Geometry check sheet. Reference: the model listing, model coordinates, mm. A direction names the side the tool comes from. Coordinates: 2 decimals unless noted, no trailing zeros. Use CSV: the item, a comma, the result in double quotes.
Autodesk Inventor part; units mm, degrees
ref_plane "YZ Plane" through (0, 0, 0) normal (1, 0, 0) x (0, 1, 0)
ref_plane "XZ Plane" through (0, 0, 0) normal (0, 1, 0) x (-1, 0, 0)
ref_plane "XY Plane" through (0, 0, 0) normal (0, 0, 1) x (1, 0, 0)
sketch "スケッチ2" plane through (0, 0, 0) normal (1, 0, 0) x (0, 1, 0)
  line L0 (0, 0) -> (-84.4498, 0)
  line L1 (-84.4498, -20) -> (1.7498, -20)
  line L2 (0, 0) -> (83.1668, 14.6646)
  line L3 (86.6398, -5.0316) -> (1.7498, -20)
  arc A0 (87.251, 14.537) -> (83.1668, 14.6646) centre (84.9033, 4.8165) ccw
  arc A1 (86.6398, -5.0316) -> (90.434, -3.5148) centre (84.9033, 4.8165) ccw
  arc A2 (-88.4498, -19.1652) -> (-84.4498, -20) centre (-84.4498, -10) ccw
  arc A3 (-84.4498, 0) -> (-88.4498, -0.8348) centre (-84.4498, -10) ccw
  arc A4 (-84.4498, -14) -> (-84.4498, -6) centre (-84.4498, -10) ccw
  line L4 (-84.4498, -6) -> (-88.4498, -6)
  line L5 (-84.4498, -14) -> (-88.4498, -14)
  line L6 (-88.4498, -0.8348) -> (-88.4498, -6)
  line L7 (-88.4498, -14) -> (-88.4498, -19.1652)
  line L8 (87.251, 14.537) -> (88.1479, 9.4503)
  line L9 (89.5371, 1.5718) -> (90.434, -3.5148)
  line L10 (1.7498, -20) -> (0, 0)
  line L11 (88.1479, 9.4503) -> (89.5371, 1.5718)
  dimension "d21" = 20
  dimension "d22" = 10
  dimension "d23" = 170
  dimension "d27" = 10
  dimension "d31" = 8
  dimension "d33" = 4
  dimension "d35" = 4
  dimension "d36" = 170
  dimension "d139" = 20
extrude "押し出し1" add sketch "スケッチ2" along normal blind 2
sketch "スケッチ4" plane through (0, 0, 0) normal (-1, 0, 0) x (0, 0, 1)
  line L0 (-20, 1.7498) -> (-5.0316, 86.6398)
  line L1 (-20, -84.4498) -> (-20, 1.7498)
  circle A0 centre (-17, -18.5891) radius 1
  circle A1 centre (-13.5138, 21.2587) radius 1
  line L2 (-17, -18.5891) -> (-13.5138, 21.2587)
  line L3 (-20, 1.7498) -> (0, 0)
  dimension "d57" = 2
  dimension "d59" = 40
  dimension "d60" = 175
  dimension "d61" = 3
  dimension "d62" = 3
hole "穴2" at (0, -18.5891, -17) at (0, 21.2587, -13.5138) direction (1, 0, 0) diameter 1.6 end through all
sketch "スケッチ6" plane through (2, 0, 0) normal (1, 0, 0) x (0, 0, -1)
  line L0 (20, 1.7498) -> (5.0316, 86.6398)
  arc A0 (5.0316, 86.6398) -> (3.5148, 90.434) centre (-4.8165, 84.9033) ccw
  line L1 (3.5148, 90.434) -> (-14.537, 87.251)
  arc A1 (-14.537, 87.251) -> (-14.6646, 83.1668) centre (-4.8165, 84.9033) ccw
  line L2 (-14.6646, 83.1668) -> (0, 0)
  line L3 (-9.3978, 53.2975) -> (-12.6117, 57.1277)
  line L4 (-14.537, 87.251) -> (-17.8212, 86.6719)
  line L5 (-17.8212, 86.6719) -> (-12.6117, 57.1277)
  line L6 (3.5148, 90.434) -> (6.799, 91.0131)
  line L7 (6.799, 91.0131) -> (12.0085, 61.4689)
  line L8 (12.0085, 61.4689) -> (10.2984, 56.7704)
  dimension "d75" = 150
  dimension "d76" = 150
  dimension "d77" = 2.5
  dimension "d78" = 2.5
  dimension "d79" = 30
extrude "押し出し2" add sketch "スケッチ6" against normal blind 2
sketch "スケッチ5" plane through (2, 0, 0) normal (1, 0, 0) x (0, 0, -1)
  line L0 (3.5148, 90.434) -> (-14.537, 87.251)
  circle A0 centre (-12.5213, 82.5293) radius 1.5
  circle A1 centre (3.2356, 85.3077) radius 1.5
  line L1 (-12.6117, 57.1277) -> (-17.8212, 86.6719)
  line L2 (-17.8212, 86.6719) -> (6.799, 91.0131)
  line L3 (6.799, 91.0131) -> (12.0085, 61.4689)
  line L4 (12.0085, 61.4689) -> (10.2984, 56.7704)
  line L5 (10.2984, 56.7704) -> (20, 1.7498)
  line L6 (20, 1.7498) -> (20, -84.4498)
  arc A2 (19.1652, -88.4498) -> (20, -84.4498) centre (10, -84.4498) ccw
  line L7 (19.1652, -88.4498) -> (14, -88.4498)
  line L8 (14, -88.4498) -> (14, -84.4498)
  arc A3 (14, -84.4498) -> (6, -84.4498) centre (10, -84.4498) ccw
  line L9 (6, -84.4498) -> (6, -88.4498)
  line L10 (6, -88.4498) -> (0.8348, -88.4498)
  arc A4 (0, -84.4498) -> (0.8348, -88.4498) centre (10, -84.4498) ccw
  line L11 (0, -84.4498) -> (0, 0)
  line L12 (0, 0) -> (-9.3978, 53.2975)
  line L13 (-9.3978, 53.2975) -> (-12.6117, 57.1277)
  circle A5 centre (17, -18.5891) radius 0.8
  circle A6 centre (13.5138, 21.2587) radius 0.8
  dimension "d70" = 5
  dimension "d71" = 5
  dimension "d72" = 3
  dimension "d114" = 16
  dimension "d123" = 4.5
hole "穴3" at (2, 82.5293, 12.5213) at (2, 85.3077, -3.2356) direction (-1, 0, 0) diameter 4 end through all
sketch "スケッチ7" plane through (2, 0, 0) normal (1, 0, 0) x (0, 0, -1)
  arc A0 (0, -84.4498) -> (0.8348, -88.4498) centre (10, -84.4498) ccw
  line L0 (0.8348, -88.4498) -> (6, -88.4498)
  circle A1 centre (3, -84.4498) radius 1
  dimension "d89" = 4
  dimension "d90" = 7
  dimension "d91" = 2
hole "穴4" at (2, -84.4498, -3) direction (-1, 0, 0) diameter 2 end through all
pattern_circular "円形状パターン3" count 5 over 180 about axis through (0, -84.4498, -10) along (-1, 0, 0) of "穴4"
sketch "スケッチ8" plane through (2, 0, 0) normal (1, 0, 0) x (0, 0, -1)
  line L0 (6.799, 91.0131) -> (-17.8212, 86.6719)
  line L1 (-17.8212, 86.6719) -> (-12.6117, 57.1277)
  circle A0 centre (-11.4794, 76.6205) radius 1.5
  circle A1 centre (4.2775, 79.3988) radius 1.5
  dimension "d102" = 11
  dimension "d103" = 11
  dimension "d104" = 16
  dimension "d105" = 4.5
  dimension "d106" = 3
hole "穴5" at (2, 76.6205, 11.4794) at (2, 79.3988, -4.2775) direction (-1, 0, 0) diameter 3.5 end through all
sketch "スケッチ11" plane through (2, 0, 0) normal (1, 0, 0) x (0, 0, -1)
  circle A0 centre (-11.4794, 76.6205) radius 1.75
  circle A1 centre (4.2775, 79.3988) radius 1.75
  line L0 (-17.8212, 86.6719) -> (-12.6117, 57.1277)
  circle A2 centre (-8.8747, 61.8483) radius 1.5
  circle A3 centre (6.8822, 64.6267) radius 1.5
  dimension "d124" = 3
  dimension "d126" = 16
  dimension "d127" = 15
  dimension "d128" = 4.5
  dimension "d130" = 15
hole "穴6" at (2, 61.8483, 8.8747) at (2, 64.6267, -6.8822) direction (-1, 0, 0) diameter 3.5 end through all
sketch "スケッチ13" plane through (2, 0, 0) normal (1, 0, 0) x (0, 0, -1)
  line L0 (0, 0) -> (0, -84.4498)
  line L1 (20, -84.4498) -> (20, 1.7498)
  line L2 (20, 1.7498) -> (10.2984, 56.7704)
  line L3 (6.799, 91.0131) -> (-17.8212, 86.6719)
  line L4 (-9.3978, 53.2975) -> (0, 0)
  line L5 (-3.8662, 44.9615) -> (9.2538, 39.6592)
  line L6 (9.2538, 39.6592) -> (6.6491, 54.4313)
  line L7 (6.6491, 54.4313) -> (-3.8662, 44.9615)
  line L8 (-2.1297, 35.1134) -> (10.9903, 29.8111)
  line L9 (10.9903, 29.8111) -> (0.475, 20.3413)
  line L10 (0.475, 20.3413) -> (-2.1297, 35.1134)
  line L11 (2.7324, 7.5388) -> (13.2477, 17.0086)
  line L12 (13.2477, 17.0086) -> (15.8525, 2.2365)
  line L13 (15.8525, 2.2365) -> (2.7324, 7.5388)
  line L14 (4, -2.2635) -> (16, -9.7635)
  line L15 (4, -17.2635) -> (4, -2.2635)
  line L16 (16, -9.7635) -> (4, -17.2635)
  line L17 (4, -30.2635) -> (16, -22.7635)
  line L18 (16, -22.7635) -> (16, -37.7635)
  line L19 (16, -37.7635) -> (4, -30.2635)
  line L20 (4, -55.2635) -> (16, -47.7635)
  line L21 (16, -47.7635) -> (4, -40.2635)
  line L22 (4, -40.2635) -> (4, -55.2635)
  line L23 (4, -65.2635) -> (16, -57.7635)
  line L24 (16, -57.7635) -> (16, -72.7635)
  line L25 (16, -72.7635) -> (4, -65.2635)
  dimension "d141" = 15
  dimension "d144" = 4
  dimension "d145" = 36
  dimension "d146" = 12
  dimension "d147" = 4
  dimension "d149" = 4
  dimension "d160" = 4
  dimension "d162" = 61
  dimension "d163" = 74
  dimension "d164" = 12
  dimension "d165" = 13
  dimension "d166" = 4
  dimension "d167" = 4
  dimension "d168" = 10
  dimension "d169" = 4
  dimension "d170" = 10
extrude "押し出し4" cut sketch "スケッチ13" against normal blind 2
fillet "フィレット1" radius 2 21 edges at (1, -65.2635, -4) (1, -30.2635, -4) (1, 44.9615, 3.8662) (1, 7.5388, -2.7324) (1, 35.1134, 2.1297) (1, -2.2635, -4) (1, -40.2635, -4) (1, 54.4313, -6.6491) (1, 17.0086, -13.2477) (1, -22.7635, -16) (1, -57.7635, -16) (1, -55.2635, -4) (1, -17.2635, -4) (1, 20.3413, -0.475) (1, 39.6592, -9.2538) (1, 2.2365, -15.8525) (1, 29.8111, -10.9903) (1, -9.7635, -16) (1, -47.7635, -16) (1, -37.7635, -16) (1, -72.7635, -16)
properties part number "Arm_Link_1" material "アルミニウム 6061"
1. Section check A-A, the plane x = 0.7. Count the separate pieces of the cut face and the enclosed holes in it, plus the area to 3 significant figures.
The answers:
separate pieces,"1"
enclosed holes,"20"
area,"3,020 mm^2"
2. Gauge pin test, flat ends, axial feed: P1, Ø1, axis at x = 0.5, y = -29.5, coming from the +Z side; P2, Ø3.5, axis at y = 82.53, z = 12.52, coming from the -X side; P3, Ø1, axis at x = 1, y = -86.5, coming from the +Z side. Record the tip position at first contact, or that the pin passes through.
The answers:
P1,"z = 0"
P2,"through"
P3,"z = -0.12"
3. Thickness scan on line 1 (Y direction, x = 0.8, z = 11.5); line 2 (Z direction, x = 1.45, y = -66.5); line 3 (Z direction, x = 0.9, y = -17). Record the ranges inside material, lowest first. Write a range as [from, to].
The answers:
line 1,"[55.8, 74.87], [78.37, 80.81], [84.25, 87.79]"
line 2,"[-20, -16], [-6.2, 0]"
line 3,"[-20, 0]"
4. Set-up check for faces 5 (the flat face through (0.99, 29.65, -15.08)), 6 (the flat face through (1.014, 72.107, 15.253)), 7 (the flat face through (1.01, -68.93, -9.87)): record each of +Z, -Z, +X, -X, +Y, -Y from which the full face is reachable in a straight line by a thin tool's end or side.
The answers:
face 5,"-Z, +X, -X"
face 6,"+Z, +X, -X, -Y"
face 7,"+X, -X"
5. Release check for a two-part mould opening along Y. For faces 1 (the flat face through (0, 0, -5)), 2 (the flat face through (0.986, 26.276, 4.633)), 3 (the flat face through (1.01, -61.65, -9.78)), 4 (the flat face through (1.014, 25.247, -5.923)) record: +Y half, -Y half, draft (parallel to the pull), parting line (faces both ways), or undercut.
The answers:
face 1,"draft"
face 2,"-Y half"
face 3,"undercut"
face 4,"undercut"
